```python
from build123d import *

# Parameters (mm, degrees)
F0_R     = 45.212
F1_DEPTH = 13.335
F2_R     = 2.5908
F3_DEPTH = 25.4
F4_R     = 14.5415
F5_DEPTH = 25.4
F6_R     = 6.731
F7_DEPTH = 10.795


with BuildPart() as f1:
    # F0 (on Top) → F1 (new body)
    with BuildSketch(Plane.XY):
        Circle(F0_R)
    extrude(amount=F1_DEPTH)

    # F2 (on face) → F3 (cut)
    with BuildSketch(Plane.XY.offset(13.335)):
        with Locations((-6.163129, 23.001109)):
            Circle(F2_R)
        with Locations((-23.001109, 6.163129)):
            Circle(F2_R)
        with Locations((-16.83798, -16.83798)):
            Circle(F2_R)
        with Locations((6.163129, -23.001109)):
            Circle(F2_R)
        with Locations((23.001109, -6.163129)):
            Circle(F2_R)
        with Locations((16.83798, 16.83798)):
            Circle(F2_R)
    extrude(amount=-F3_DEPTH, mode=Mode.SUBTRACT)

    # F4 (on face) → F5 (cut)
    with BuildSketch(Plane.XY.offset(13.335)):
        Circle(F4_R)
    extrude(amount=-F5_DEPTH, mode=Mode.SUBTRACT)

    # F6 (on face) → F7 (cut)
    with BuildSketch(Plane.XY.offset(13.335)):
        with Locations((-6.163129, 23.001109)):
            Circle(F6_R)
        with Locations((16.83798, 16.83798)):
            Circle(F6_R)
        with Locations((23.001109, -6.163129)):
            Circle(F6_R)
        with Locations((6.163129, -23.001109)):
            Circle(F6_R)
        with Locations((-16.83798, -16.83798)):
            Circle(F6_R)
        with Locations((-23.001109, 6.163129)):
            Circle(F6_R)
    extrude(amount=-F7_DEPTH, mode=Mode.SUBTRACT)


solid = f1.part
```
Could you check a few things on this model? Use its own coordinates, in mm. A direction names the side the tool comes from. Coordinates: 2 decimals unless noted, no trailing zeros. Write each loop counter-clockwise with the first axis right and the second up, starting at its lowest first coordinate (ties: lowest second). Pieces come first, ordered by that corner, then holes. Notation, with made-up numbers: (-38.5, 52.5) -> (-1.5, 52.5) arc R12 cw to (-1.5, 56.5) -> close; hole circle Ø10 at (18, 88). An arc over 180 degrees is marked (long way). Return JSON: item names as keys, results as strings.
(1) Which directions (+Z, -Z, +X, -X, +Y, -Y) give clear straight access to the entire face, cutting with the end or side of a thin tool? Please do faces 1 (the cylindrical face through (26.107, -12.135, 8.013)), 2 (the cylindrical face through (-10.718, 9.828, 6.761)).
Numbers:
{"face 1": "+Z", "face 2": "+Z, -Z"}
(2) Imagine slicing it at C-C, the plane y = -18. Please give me the cut outline in (x, z) (3 decimals), then the cut area to 3 significant figures.
Numbers:
{"outline": "(-41.474, 0) -> (-19.154, 0) -> (-19.154, 2.54) -> (-23.468, 2.54) -> (-23.468, 13.335) -> (-41.474, 13.335) -> close; (-14.522, 0) -> (41.474, 0) -> (41.474, 13.335) -> (10.668, 13.335) -> (10.668, 2.54) -> (1.658, 2.54) -> (1.658, 13.335) -> (-10.208, 13.335) -> (-10.208, 2.54) -> (-14.522, 2.54) -> close", "area": "854 mm2"}
(3) I need wall thicknesses on L1, parallel to X at y = -12, z = 5; L2, parallel to X at y = -13.5, z = 6.75; L3, parallel to Y at x = 21, z = 12.75. Which ranges of each line are inside material? Lowest first, please.
Numbers:
{"L1": "x = -43.59 to -21.52, -12.16 to -8.21, 8.21 to 19.65, 26.35 to 43.59", "L2": "x = -43.15 to -22.68, -10.99 to -5.4, 5.4 to 43.15", "L3": "y = -40.04 to -12.59, 0.26 to 11.55, 22.13 to 40.04"}
(4) I'm going to push flat-ended pins straight in: pin 1 (6 mm diameter, centred on x = 4.5, z = 10.5, fed in from +Y); pin 2 (5 mm diameter, centred on x = 18, z = 6, fed in from +Y); pin 3 (8 mm diameter, centred on y = 22, z = 10, fed in from +X); pin 4 (4 mm diameter, centred on x = -23, y = 6.16, fed in from +Z). Where does each tip first touch, or does it pass through?
Numbers:
{"pin 1": "stops at y = 45.19", "pin 2": "stops at y = 42.47", "pin 3": "stops at x = 41.47", "pin 4": "passes through"}
(5) Imagine slicing it at B-B, the plane z = 1.5. Please give me the cut outline in (x, y).
Numbers:
{"outline": "circle Ø90.42 at (0, 0); hole circle Ø5.18 at (-23, 6.16); hole circle Ø5.18 at (-16.84, -16.84); hole circle Ø29.08 at (0, 0); hole circle Ø5.18 at (-6.16, 23); hole circle Ø5.18 at (6.16, -23); hole circle Ø5.18 at (16.84, 16.84); hole circle Ø5.18 at (23, -6.16)"}
(6) Imagine slicing it at A-A, the plane x = -5.5. Please give me the cut outline in (y, z) (3 decimals), then the cut area to 4 significant figures.
Numbers:
{"outline": "(-44.876, 0) -> (-13.461, 0) -> (-13.461, 13.335) -> (-44.876, 13.335) -> close; (13.461, 0) -> (20.497, 0) -> (20.497, 2.54) -> (16.303, 2.54) -> (16.303, 13.335) -> (13.461, 13.335) -> close; (25.506, 0) -> (44.876, 0) -> (44.876, 13.335) -> (29.699, 13.335) -> (29.699, 2.54) -> (25.506, 2.54) -> close", "area": "680.5 mm2"}
